Check sheet for the modelled part. Datum: model origin and axes. Units: mm. Face numbers are marked on the shaded views. A direction names the side the tool comes from. Give positions to 0.01 mm unless a question says otherwise; leave off trailing zeros. Write each loop counter-clockwise with the first axis right and the second up, starting at its lowest first coordinate (ties: lowest second). Pieces come first, ordered by that corner, then holes. Notation, with made-up numbers: (-24.5, 71.5) -> (32.5, 71.5) arc R19 cw to (32.5, 77.5) -> close; hole circle Ø4 at (40.25, 64). An arc over 180 degrees is marked (long way). Answer as a JSON object with one key per item and string values.
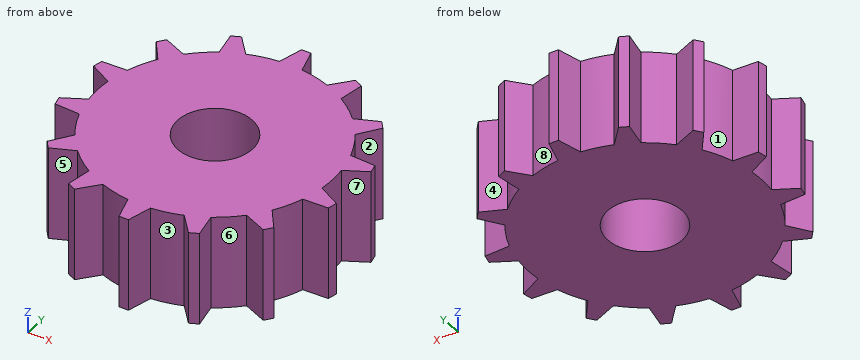
from build123d import *

# Parameters (mm, degrees)
ESQUISSE2_R        = 4
BOSS_EXTRU_1_DEPTH = 10


with BuildPart() as part:
    # Esquisse2 → Boss.-Extru.1 (new body)
    with BuildSketch(Plane.XY):
        with BuildLine():
            ThreePointArc((-19.500069449, 14.991666667), (-20, 15), (-20.499930551, 14.991666667))
            Line((-20.499930551, 14.991666667), (-21.2, 12.442266675))
            ThreePointArc((-21.2, 12.442266675), (-22.781511674, 12.186598902), (-24.317334546, 11.730755407))
            Line((-24.317334546, 11.730755407), (-26.054218527, 13.723936681))
            ThreePointArc((-26.054218527, 13.723936681), (-26.508256087, 13.514533019), (-26.955062251, 13.290113208))
            Line((-26.955062251, 13.290113208), (-26.479659829, 10.689434433))
            ThreePointArc((-26.479659829, 10.689434433), (-27.793622523, 9.772893531), (-28.979568037, 8.695824163))
            Line((-28.979568037, 8.695824163), (-31.409255375, 9.738012723))
            ThreePointArc((-31.409255375, 9.738012723), (-31.727472237, 9.352347028), (-32.032658575, 8.956289836))
            Line((-32.032658575, 8.956289836), (-30.475943562, 6.819428605))
            ThreePointArc((-30.475943562, 6.819428605), (-31.262110849, 5.423546739), (-31.863287951, 3.938578296))
            Line((-31.863287951, 3.938578296), (-34.50454927, 3.823355916))
            ThreePointArc((-34.50454927, 3.823355916), (-34.623918683, 3.337814009), (-34.727039297, 2.84856342))
            Line((-34.727039297, 2.84856342), (-32.397338193, 1.598751306))
            ThreePointArc((-32.397338193, 1.598751306), (-32.5, 0), (-32.397338193, -1.598751306))
            Line((-32.397338193, -1.598751306), (-34.727039297, -2.84856342))
            ThreePointArc((-34.727039297, -2.84856342), (-34.623918683, -3.337814009), (-34.50454927, -3.823355916))
            Line((-34.50454927, -3.823355916), (-31.863287951, -3.938578296))
            ThreePointArc((-31.863287951, -3.938578296), (-31.262110849, -5.423546739), (-30.475943562, -6.819428605))
            Line((-30.475943562, -6.819428605), (-32.032658575, -8.956289836))
            ThreePointArc((-32.032658575, -8.956289836), (-31.727472237, -9.352347028), (-31.409255375, -9.738012723))
            Line((-31.409255375, -9.738012723), (-28.979568037, -8.695824163))
            ThreePointArc((-28.979568037, -8.695824163), (-27.793622523, -9.772893531), (-26.479659829, -10.689434433))
            Line((-26.479659829, -10.689434433), (-26.955062251, -13.290113208))
            ThreePointArc((-26.955062251, -13.290113208), (-26.508256087, -13.514533019), (-26.054218527, -13.723936681))
            Line((-26.054218527, -13.723936681), (-24.317334546, -11.730755407))
            ThreePointArc((-24.317334546, -11.730755407), (-22.781511674, -12.186598902), (-21.2, -12.442266675))
            Line((-21.2, -12.442266675), (-20.499930551, -14.991666667))
            ThreePointArc((-20.499930551, -14.991666667), (-20, -15), (-19.500069449, -14.991666667))
            Line((-19.500069449, -14.991666667), (-18.8, -12.442266675))
            ThreePointArc((-18.8, -12.442266675), (-17.218488326, -12.186598902), (-15.682665454, -11.730755407))
            Line((-15.682665454, -11.730755407), (-13.945781473, -13.723936681))
            ThreePointArc((-13.945781473, -13.723936681), (-13.491743913, -13.514533019), (-13.044937749, -13.290113208))
            Line((-13.044937749, -13.290113208), (-13.520340171, -10.689434433))
            ThreePointArc((-13.520340171, -10.689434433), (-12.206377477, -9.772893531), (-11.020431963, -8.695824163))
            Line((-11.020431963, -8.695824163), (-8.590744625, -9.738012723))
            ThreePointArc((-8.590744625, -9.738012723), (-8.272527763, -9.352347028), (-7.967341425, -8.956289836))
            Line((-7.967341425, -8.956289836), (-9.524056438, -6.819428605))
            ThreePointArc((-9.524056438, -6.819428605), (-8.737889151, -5.423546739), (-8.136712049, -3.938578296))
            Line((-8.136712049, -3.938578296), (-5.49545073, -3.823355916))
            ThreePointArc((-5.49545073, -3.823355916), (-5.376081317, -3.337814009), (-5.272960703, -2.84856342))
            Line((-5.272960703, -2.84856342), (-7.602661807, -1.598751306))
            ThreePointArc((-7.602661807, -1.598751306), (-7.5, 0), (-7.602661807, 1.598751306))
            Line((-7.602661807, 1.598751306), (-5.272960703, 2.84856342))
            ThreePointArc((-5.272960703, 2.84856342), (-5.376081317, 3.337814009), (-5.49545073, 3.823355916))
            Line((-5.49545073, 3.823355916), (-8.136712049, 3.938578296))
            ThreePointArc((-8.136712049, 3.938578296), (-8.737889151, 5.423546739), (-9.524056438, 6.819428605))
            Line((-9.524056438, 6.819428605), (-7.967341425, 8.956289836))
            ThreePointArc((-7.967341425, 8.956289836), (-8.272527763, 9.352347028), (-8.590744625, 9.738012723))
            Line((-8.590744625, 9.738012723), (-11.020431963, 8.695824163))
            ThreePointArc((-11.020431963, 8.695824163), (-12.206377477, 9.772893531), (-13.520340171, 10.689434433))
            Line((-13.520340171, 10.689434433), (-13.044937749, 13.290113208))
            ThreePointArc((-13.044937749, 13.290113208), (-13.491743913, 13.514533019), (-13.945781473, 13.723936681))
            Line((-13.945781473, 13.723936681), (-15.682665454, 11.730755407))
            ThreePointArc((-15.682665454, 11.730755407), (-17.218488326, 12.186598902), (-18.8, 12.442266675))
            Line((-18.8, 12.442266675), (-19.500069449, 14.991666667))
        make_face()
        with Locations((-20, 0)):
            Circle(ESQUISSE2_R, mode=Mode.SUBTRACT)
    extrude(amount=BOSS_EXTRU_1_DEPTH)


solid = part.part
1. Access from +Z, -Z, +X, -X, +Y, -Y to the whole of each face (thin tool, end or side, straight path). Record for the marked faces 1, 2, 3 and 4.
Determined:
{"face 1": "+Z, -Z, -X", "face 2": "+Z, -Z, +X", "face 3": "+Z, -Z, -Y", "face 4": "+Z, -Z, +Y"}
2. Sectioned sample at D-D, the plane x = -29.5. Enter the section's corners in (y, z), plus the area to 3 significant figures.
Determined:
{"outline": "(-8.92, 0) -> (8.92, 0) -> (8.92, 10) -> (-8.92, 10) -> close", "area": "178 mm^2"}
3. Sectioned sample at B-B, the plane y = 0. Enter the section's corners in (x, z), plus the area to 3 significant figures.
Determined:
{"outline": "(-32.5, 0) -> (-24, 0) -> (-24, 10) -> (-32.5, 10) -> close; (-16, 0) -> (-7.5, 0) -> (-7.5, 10) -> (-16, 10) -> close", "area": "170 mm^2"}
4. Sectioned sample at A-A, the plane x = -20. Enter the section's corners in (y, z).
Determined:
{"outline": "(-15, 0) -> (-4, 0) -> (-4, 10) -> (-15, 10) -> close; (4, 0) -> (15, 0) -> (15, 10) -> (4, 10) -> close"}
5. Scan lines: L1, parallel to Y at x = -20, z = 3; L2, parallel to X at y = 12.75, z = 1.25; L3, parallel to X at y = -12.5, z = 4.75. Record each from-to range of solid material in increasing order. Write a range as [from, to].
Determined:
{"L1": "[-15, -4], [4, 15]", "L2": "[-26.86, -25.21], [-21.12, -18.88], [-14.79, -13.14]", "L3": "[-26.81, -24.99], [-21.18, -18.82], [-15.01, -13.19]"}
6. Mould release check, pull along Y, two halves, no side actions. Record for the marked faces 5, 6, 7 and 8: released by +Y, released by -Y, zero draft, split by the parting line, or undercut.
Determined:
{"face 5": "released by -Y", "face 6": "undercut", "face 7": "undercut", "face 8": "released by +Y"}
7. Go/stop test with flat-tipped pins: P1, Ø3, axis at x = -10, z = 1.5, coming from the +Y side; P2, Ø4, axis at x = -27, z = 6.5, coming from the -Y side; P3, Ø3, axis at y = -7.5, z = 3, coming from the +X side. Record where each tip stops, or that it passes through.
Determined:
{"P1": "y = 9.74", "P2": "y = -13.72", "P3": "x = -7.97"}
8. Sectioned sample at C-C, the plane y = -4.75. Enter the section's corners in (x, z), plus the area to 3 significant figures.
Determined:
{"outline": "(-31.56, 0) -> (-8.44, 0) -> (-8.44, 10) -> (-31.56, 10) -> close", "area": "231 mm^2"}
